Check sheet for the modelled part. Datum: model origin and axes. Units: mm. A direction names the side the tool comes from. Give positions to 0.01 mm unless a question says otherwise; leave off trailing zeros. Write each loop counter-clockwise with the first axis right and the second up, starting at its lowest first coordinate (ties: lowest second). Pieces come first, ordered by that corner, then holes. Notation, with made-up numbers: M 78.25,1 L 107.25,1 A12 ccw 107.25,24 Z; hole C 59,-8 d4. An arc over 180 degrees is marked long. Write item = value, one per line. Start each with the question number.
1) Sectioned sample at C-C, the plane x = 50. Count the separate pieces of the cut face and the enclosed holes in it, then the cut area to 3 significant figures.
2) Sectioned sample at B-B, the plane y = -107.5. Record the cut outline in (x, z), then the cut area to 3 significant figures.
3) Gauge pin test, flat ends, axial feed: pin 1 (12.5 mm diameter, centred on y = -108, z = -38, fed in from +X); pin 2 (4 mm diameter, centred on x = 34, y = 2, fed in from -Z); pin 3 (9 mm diameter, centred on x = 50, y = -25, fed in from +Z); pin 4 (12 mm diameter, centred on y = -18, z = -21.5, fed in from -X). Record the tip position at first contact, or that the pin passes through.
4) Scan lines: L1, parallel to Z at x = 39.5, y = -48.5; L2, parallel to X at y = -83.5, z = -49; L3, parallel to X at y = -104, z = -12. Record each from-to range of solid material in increasing order.
5) Draft check along Z on faces 1 (the face through (50, -20, -58)), 2 (the face through (2, -5, -55)), 3 (the face through (95, -72, -41)). Enter one of: pulls with the +Z half, pulls with the -Z half, needs draft (parallel to the pull), parting line crosses it, or undercut.
6) Set-up check for faces 4 (the face through (49, 0, -25)), 5 (the face through (100, -36, -34)), 6 (the face through (50, -37, -60)), 7 (the face through (97.5, -59.2, -5)), 8 (the face through (50, -15, -58)): record each of +Z, -Z, +X, -X, +Y, -Y from which the full face is reachable in a straight line by a thin tool's end or side.
Autodesk Inventor part; units mm, degrees
ref_plane "YZ Plane" through (0, 0, 0) normal (1, 0, 0) x (0, 1, 0)
ref_plane "XZ Plane" through (0, 0, 0) normal (0, 1, 0) x (-1, 0, 0)
ref_plane "XY Plane" through (0, 0, 0) normal (0, 0, 1) x (1, 0, 0)
sketch "Esquisse1" plane through (0, 0, 0) normal (0, 0, 1) x (1, 0, 0)
  line L0 (0, 0) -> (100, 0)
  line L1 (100, 0) -> (100, -50)
  line L2 (100, -50) -> (0, -50)
  line L3 (0, -50) -> (0, 0)
  dimension "d0" = 50
  dimension "d1" = 100
extrude "Extrusion1" add sketch "Esquisse1" along normal blind 5
sketch "Esquisse2" plane through (0, 0, 5) normal (0, 0, 1) x (1, 0, 0)
  line L0 (100, 0) -> (0, 0) construction
  line L1 (0, -50) -> (100, -50) construction
  line L2 (0, 0) -> (100, -50) construction
  line L3 (0, 0) -> (0, -50) construction
  line L4 (100, 0) -> (0, -50) construction
  circle A0 centre (50, -25) radius 5
  dimension "d4" = 10
extrude "Extrusion2" cut sketch "Esquisse2" against normal blind 5
sketch "Esquisse3" plane through (0, 0, 0) normal (0, 0, -1) x (-1, 0, 0)
  line L0 (-100, 0) -> (-95, 0)
  line L1 (-95, 0) -> (-95, -50)
  line L2 (-95, -50) -> (-100, -50)
  line L3 (-100, -50) -> (-100, 0)
  line L4 (0, 0) -> (-5, 0)
  line L5 (-5, 0) -> (-5, -50)
  line L6 (-5, -50) -> (0, -50)
  line L7 (0, -50) -> (0, 0)
  dimension "d7" = 5
  dimension "d8" = 5
extrude "Extrusion3" add sketch "Esquisse3" along normal blind 60
chamfer "Chanfrein1" distance 10 angle 45 1 edges at (97.5, 0, -60)
chamfer "Chanfrein2" distance 10 angle 45 1 edges at (2.5, 0, -60)
sketch "Esquisse4" plane through (100, -50, 5) normal (1, 0, 0) x (0, 0, -1)
  line L0 (0, 0) -> (15, -27.5984)
  line L1 (0, 50) -> (0, 0)
  line L2 (0, 0) -> (15, 0)
  line L3 (0, 0) -> (65, 0)
  line L4 (65, 0) -> (65, -70)
  line L5 (65, -70) -> (15, -70)
  line L6 (15, -27.5984) -> (15, -70)
  point P0 (5, 50)
  dimension "d17" = 15
  dimension "d18" = 70
extrude "Extrusion4" add sketch "Esquisse4" against normal blind 5
sketch "Esquisse5" plane through (100, 0, 5) normal (1, 0, 0) x (0, 0, -1)
  line L0 (65, -120) -> (15, -120)
  line L1 (65, -10) -> (65, -120)
  line L2 (15, -120) -> (65, -120)
  line L3 (65, -120) -> (65, -95)
  line L4 (65, -95) -> (15, -95)
  line L5 (15, -95) -> (15, -120)
  point P0 (5, 0)
  dimension "d21" = 25
extrude "Extrusion5" cut sketch "Esquisse5" against normal blind 2.5
sketch "Esquisse6" plane through (97.5, 0, 5) normal (1, 0, 0) x (0, 0, -1)
  circle A0 centre (25, -107.5) radius 2.6
  circle A1 centre (55, -107.5) radius 2.6
  line L0 (15, -120) -> (15, -95)
  line L1 (65, -95) -> (65, -120)
  line L2 (15, -95) -> (65, -95)
  point P0 (5, 0)
  dimension "d24" = 5.2
  dimension "d25" = 5.2
  dimension "d26" = 10
  dimension "d27" = 10
  dimension "d28" = 12.5
  dimension "d29" = 12.5
extrude "Extrusion6" cut sketch "Esquisse6" against normal blind 2.5
sketch "Esquisse8" plane through (0, 0, 5) normal (0, 1, 0) x (1, 0, 0)
  line L0 (3.5, 3.5) -> (96.5, 3.5)
  line L1 (96.5, 3.5) -> (96.5, 55)
  line L2 (96.5, 55) -> (3.5, 55)
  line L3 (3.5, 55) -> (3.5, 3.5)
  point P0 (0, 5)
extrude "Extrusion8" add sketch "Esquisse8" along normal blind 5
chamfer "Chanfrein5" distance 3.5 angle 45 1 edges at (96.5, 0, -24.25)
chamfer "Chanfrein6" distance 3.5 angle 45 1 edges at (50, 0, 1.5)
chamfer "Chanfrein7" distance 3.5 angle 45 1 edges at (3.5, 0, -24.25)
sketch "Esquisse9" plane through (0, 0, -60) normal (0, 0, -1) x (-1, 0, 0)
  line L0 (-5, -50) -> (0, -50)
  line L1 (-95, -10) -> (-95, 0)
  line L2 (-5, -50) -> (-95, -50)
  line L3 (-95, -50) -> (-95, -10)
  line L4 (-95, -10) -> (-5, -10)
  line L5 (-5, -10) -> (-5, -50)
  point P0 (0, 0)
extrude "Extrusion9" add sketch "Esquisse9" against normal blind 5
sketch "Esquisse10" plane through (0, -50, -60) normal (-1, 0, 0) x (0, 0, 1)
  line L0 (50, -27.5984) -> (65, 0)
  line L1 (65, 0) -> (50, -27.5984)
  line L2 (50, -70) -> (50, -27.5984)
  line L3 (50, -27.5984) -> (50, -70)
  line L4 (0, -70) -> (50, -70)
  line L5 (50, -70) -> (0, -70)
  line L6 (0, -70) -> (0, 0)
  line L7 (0, 0) -> (65, 0)
  point P0 (60, 50)
extrude "Extrusion10" add sketch "Esquisse10" against normal blind 5
sketch "Esquisse11" plane through (0, 0, -50) normal (-1, 0, 0) x (0, 0, 1)
  line L0 (40, -77.5984) -> (40, -120)
  line L1 (-10, -120) -> (40, -120)
  line L2 (40, -120) -> (40, -95)
  line L3 (40, -95) -> (-10, -95)
  line L4 (-10, -95) -> (-10, -120)
  point P0 (50, 0)
  dimension "d63" = 25
extrude "Extrusion11" cut sketch "Esquisse11" against normal blind 2.5
sketch "Esquisse12" plane through (2.5, 0, -50) normal (-1, 0, 0) x (0, 0, 1)
  circle A0 centre (0, -107.5) radius 2.6
  circle A1 centre (0, -107.5) radius 2.6
  circle A2 centre (30, -107.5) radius 2.6
  circle A3 centre (30, -107.5) radius 2.6
  point P0 (50, 0)
extrude "Extrusion12" cut sketch "Esquisse12" against normal blind 2.5
sketch "Esquisse13" plane through (100, -95, -10) normal (1, 0, 0) x (0, 0, -1)
  line L0 (-10, 90) -> (35.5969, 90)
  line L1 (-10, 47.7175) -> (-10, 90)
  line L2 (-15, 45) -> (-15, 95)
  line L3 (-15, 45) -> (0, 17.4016)
  line L4 (-10, 47.7175) -> (-10, 45)
  line L5 (-15, 45) -> (0, 17.4016)
  line L6 (-15, 95) -> (40, 95)
  line L7 (35.5969, 90) -> (40, 90)
  line L8 (45, 85) -> (45, 45)
  line L9 (45, 85) -> (45, 5.9149)
  line L10 (5, 17.4016) -> (5, 5)
  line L11 (5, 5) -> (45, 5)
  line L12 (45, 5) -> (45, 5.9149)
  line L13 (0, 0) -> (50, 0)
  line L14 (0, 17.4016) -> (0, 0)
  line L15 (5, 17.4016) -> (5, 17.4016)
  line L16 (5, 17.4016) -> (-10, 45)
  line L17 (40, 90) -> (45, 85)
  line L18 (45, 45) -> (45, 85) construction
  circle A0 centre (17.2708, 47.8542) radius 5
  circle A1 centre (17.2708, 47.8542) radius 10
  line L19 (19.4502, 57.6138) -> (40, 90)
  line L20 (45, 85) -> (25.2526, 53.8784)
  line L21 (3.6653, 19.8572) -> (15.2197, 38.0668)
  line L22 (9.3688, 41.7257) -> (-0.1053, 26.7947)
  line L23 (-5.8908, 90) -> (15.0684, 57.6086) construction
  line L24 (19.4729, 38.0996) -> (40.8908, 5)
  line L25 (-5.8908, 90) -> (15.0684, 57.6086)
  line L26 (25.2663, 41.8482) -> (45, 11.3507)
  line L27 (-10, 83.6477) -> (9.2748, 53.8594)
  line L28 (-10, 45) -> (-10, 95)
  line L29 (-10, 83.6477) -> (-10, 45)
  line L30 (-10, 45) -> (-0.1053, 26.7947)
  dimension "d71" = 5
  dimension "d72" = 5
  dimension "d73" = 5
  dimension "d74" = 5
  dimension "d78" = 5
  dimension "d79" = 10
  dimension "d83" = 5
extrude "Extrusion13" cut sketch "Esquisse13" against normal blind 5 contours L0 L7 L19 A1 L25 | L27 A1 L22 L16 L4 L1 | L8 L9 L26 A1 L20 | A1 L24 L11 L10 L16 L21 | A0
sketch "Esquisse14" plane through (0, 0, -50) normal (-1, 0, 0) x (0, 0, 1)
  line L0 (0, -5) -> (45.8908, -5)
  line L1 (0, -5) -> (45.8908, -5)
  line L2 (45.8908, -5) -> (50, -5)
  line L3 (0, -5) -> (-5, -10)
  line L4 (-5, -10) -> (-5, -90)
  line L5 (50, -5) -> (50, -50)
  line L6 (35, -77.5984) -> (35, -90)
  line L7 (50, -50) -> (35, -77.5984)
  line L8 (35, -77.5984) -> (35, -90)
  line L9 (35, -90) -> (-5, -90)
  line L10 (35, -90) -> (-0.8908, -90)
  line L11 (-5, -10) -> (14.7474, -41.1216)
  line L12 (-5, -10) -> (14.7474, -41.1216)
  line L13 (24.7803, -56.9332) -> (36.3347, -75.1428)
  line L14 (24.7803, -56.9332) -> (36.3347, -75.1428)
  line L15 (30.6312, -53.2743) -> (40.1053, -68.2053)
  line L16 (30.6312, -53.2743) -> (40.1053, -68.2053)
  arc A0 (30.6312, -53.2743) -> (30.7252, -41.1406) centre (22.7292, -47.1458) ccw
  line L17 (50, -11.3523) -> (30.7252, -41.1406)
  line L18 (-5, -83.6493) -> (14.7337, -53.1518)
  line L19 (14.7337, -53.1518) -> (-5, -83.6493)
  arc A1 (20.5271, -56.9004) -> (24.7803, -56.9332) centre (22.7292, -47.1458) ccw
  line L20 (-0.8908, -90) -> (20.5271, -56.9004)
  line L21 (-0.8908, -90) -> (20.5271, -56.9004)
  line L22 (20.5498, -37.3862) -> (0, -5)
  line L23 (0, -5) -> (20.5741, -37.4244)
  line L24 (24.9316, -37.3914) -> (45.8908, -5)
  line L25 (45.8908, -5) -> (24.9316, -37.3914)
  line L26 (-0.8908, -90) -> (35, -90)
  line L27 (35, -77.5984) -> (36.3347, -75.1428)
  line L28 (-5, -50) -> (-5, -10)
  line L29 (-5, -10) -> (14.7474, -41.1216)
  line L30 (-5, -10) -> (-5, -83.6493)
  arc A2 (14.7474, -41.1216) -> (14.7337, -53.1518) centre (22.7292, -47.1458) ccw
  line L31 (-5, -83.6493) -> (14.7337, -53.1518)
  line L32 (0, -5) -> (20.5741, -37.4244)
  line L33 (0, -5) -> (45.8908, -5)
  arc A3 (24.9316, -37.3914) -> (20.5498, -37.3862) centre (22.7292, -47.1458) ccw
  line L34 (24.9316, -37.3914) -> (45.8908, -5)
  line L35 (40.1053, -68.2053) -> (30.6312, -53.2743)
  line L36 (50, -50) -> (40.1053, -68.2053)
  line L37 (40.1053, -68.2053) -> (50, -50)
  line L38 (30.7252, -41.1406) -> (50, -11.3523)
  line L39 (50, -50) -> (50, -11.3523)
  line L40 (50, -11.3523) -> (30.7252, -41.1406)
  circle A4 centre (22.7292, -47.1458) radius 5
extrude "Extrusion14" cut sketch "Esquisse14" against normal blind 5 contours L0 L24 A3 L22 | L11 A2 L18 L4 | L5 L7 L15 A0 L17 | L20 A1 L13 L7 L6 L9 | A4
sketch "Esquisse15" plane through (0, 0, -60) normal (0, 0, -1) x (-1, 0, 0)
  line L0 (-5, -50) -> (-95, -50) construction
  circle A0 centre (-50, -30) radius 5
  circle A1 centre (-50, -30) radius 10
  line L1 (-95, -10) -> (-5, -10) construction
  line L2 (-95, -10) -> (-95, -50) construction
  line L3 (-5, -9.9768) -> (-5, -50) construction
  line L4 (-90, -18.6348) -> (-90, -45)
  line L5 (-90, -45) -> (-10, -45)
  line L6 (-10, -45) -> (-10, -15)
  line L7 (-10, -15) -> (-90, -15)
  line L8 (-90, -15) -> (-90, -18.6348)
  line L9 (-90, -15) -> (-59.6422, -27.3489)
  line L10 (-83.75, -15) -> (-58.7548, -25.1675)
  line L11 (-41.2507, -25.1575) -> (-16.2956, -15)
  line L12 (-10, -15) -> (-40.3559, -27.3558)
  line L13 (-10, -45) -> (-40.3578, -32.6511)
  line L14 (-16.25, -45) -> (-41.2452, -34.8325)
  line L15 (-83.7044, -45) -> (-58.7493, -34.8425)
  line L16 (-90, -45) -> (-59.6441, -32.6442)
  point P0 (0, 0)
  dimension "d90" = 20
  dimension "d89" = 10
  dimension "d91" = 5
  dimension "d92" = 5
  dimension "d93" = 5
  dimension "d94" = 5
extrude "Extrusion15" cut sketch "Esquisse15" against normal blind 5 contours A0 | A1 L12 L6 L13 | A1 L10 L7 L11 | L14 L5 L15 A1 | A1 L16 L4 L8 L9
properties part number "Biceps1 v2" material "Plastique ABS"
Data:
q1.separate_pieces = 6
q1.enclosed_holes = 0
q1.area = 564 mm2
q2.outline = M 2.5,-60 L 5,-60 L 5,-52.6 L 2.5,-52.6 Z; M 2.5,-47.4 L 5,-47.4 L 5,-22.6 L 2.5,-22.6 Z; M 2.5,-17.4 L 5,-17.4 L 5,-10 L 2.5,-10 Z; M 95,-60 L 97.5,-60 L 97.5,-52.6 L 95,-52.6 Z; M 95,-47.4 L 97.5,-47.4 L 97.5,-22.6 L 95,-22.6 Z; M 95,-17.4 L 97.5,-17.4 L 97.5,-10 L 95,-10 Z
q2.area = 198 mm2
q3.pin_1 = 97.5
q3.pin_2 = -50
q3.pin_3 = -55
q3.pin_4 = through
q4.L1 = -60 to -55, 0 to 5
q4.L2 = 0 to 5, 95 to 100
q4.L3 = 2.5 to 5, 95 to 97.5
q5.face_1 = needs draft
q5.face_2 = pulls with the -Z half
q5.face_3 = undercut
q6.face_4 = -Z, -Y
q6.face_5 = +Z, -Z, +X, +Y, -Y
q6.face_6 = -Z, +X, -X, +Y, -Y
q6.face_7 = +X, -X
q6.face_8 = -Z
